```python
from build123d import *

# Parameters (mm, degrees)
SKETCH1_R           = 0.85
BOSS_EXTRUDE1_DEPTH = 3


with BuildPart() as part:
    # Sketch1 → Boss-Extrude1 (new body)
    with BuildSketch(Plane.XY):
        with BuildLine():
            Line((2.012075091, 4.025115381), (3.394482569, 4.82324871))
            Line((3.394482569, 4.82324871), (4.160527012, 4.1804611))
            Line((4.160527012, 4.1804611), (3.614571661, 2.6804611))
            ThreePointArc((3.614571661, 2.6804611), (3.897114317, 2.25), (4.128633237, 1.790080332))
            Line((4.128633237, 1.790080332), (5.700649018, 1.512891535))
            Line((5.700649018, 1.512891535), (5.874297196, 0.528083782))
            Line((5.874297196, 0.528083782), (4.491889718, -0.270049547))
            ThreePointArc((4.491889718, -0.270049547), (4.431634889, -0.7814168), (4.313358007, -1.282553199))
            Line((4.313358007, -1.282553199), (5.339418436, -2.505364402))
            Line((5.339418436, -2.505364402), (4.839418436, -3.371389806))
            Line((4.839418436, -3.371389806), (3.267402655, -3.09420101))
            ThreePointArc((3.267402655, -3.09420101), (2.892544244, -3.447199994), (2.479814627, -3.755065834))
            Line((2.479814627, -3.755065834), (2.479814627, -5.351332492))
            Line((2.479814627, -5.351332492), (1.540122006, -5.693352636))
            Line((1.540122006, -5.693352636), (0.514061576, -4.470541432))
            ThreePointArc((0.514061576, -4.470541432), (0, -4.5), (-0.514061576, -4.470541432))
            Line((-0.514061576, -4.470541432), (-1.540122006, -5.693352636))
            Line((-1.540122006, -5.693352636), (-2.479814627, -5.351332492))
            Line((-2.479814627, -5.351332492), (-2.479814627, -3.755065834))
            ThreePointArc((-2.479814627, -3.755065834), (-2.892544244, -3.447199994), (-3.267402655, -3.09420101))
            Line((-3.267402655, -3.09420101), (-4.839418436, -3.371389806))
            Line((-4.839418436, -3.371389806), (-5.339418436, -2.505364402))
            Line((-5.339418436, -2.505364402), (-4.313358007, -1.282553199))
            ThreePointArc((-4.313358007, -1.282553199), (-4.431634889, -0.7814168), (-4.491889718, -0.270049547))
            Line((-4.491889718, -0.270049547), (-5.874297196, 0.528083782))
            Line((-5.874297196, 0.528083782), (-5.700649018, 1.512891535))
            Line((-5.700649018, 1.512891535), (-4.128633237, 1.790080332))
            ThreePointArc((-4.128633237, 1.790080332), (-3.897114317, 2.25), (-3.614571661, 2.6804611))
            Line((-3.614571661, 2.6804611), (-4.160527012, 4.1804611))
            Line((-4.160527012, 4.1804611), (-3.394482569, 4.82324871))
            Line((-3.394482569, 4.82324871), (-2.012075091, 4.025115381))
            ThreePointArc((-2.012075091, 4.025115381), (-1.539090645, 4.228616794), (-1.045955351, 4.376754209))
            Line((-1.045955351, 4.376754209), (-0.5, 5.876754209))
            Line((-0.5, 5.876754209), (0.5, 5.876754209))
            Line((0.5, 5.876754209), (1.045955351, 4.376754209))
            ThreePointArc((1.045955351, 4.376754209), (1.539090645, 4.228616794), (2.012075091, 4.025115381))
        make_face()
        Circle(SKETCH1_R, mode=Mode.SUBTRACT)
    extrude(amount=BOSS_EXTRUDE1_DEPTH)


solid = part.part
```
Model file for the job. Use its own axes, mm. A direction names the side the tool comes from. Round coordinates to 2 decimals unless told otherwise and drop trailing zeros. Write each loop counter-clockwise with the first axis right and the second up, starting at its lowest first coordinate (ties: lowest second). Pieces come first, ordered by that corner, then holes. Notation, with made-up numbers: (71.5, 83) - (127.5, 83) arc R16 ccw to (127.5, 112) - close; hole circle Ø1 at (9.25, 63). An arc over 180 degrees is marked (long way). Use CSV: the item, a comma, the result in double quotes. Start each with the question number.
Item 1: Band-saw the part on B-B (y = 0). Write the cut outline in (x, z), and give its area (3 significant figures).
Item 2: Two-plate mould, pull along Y, no slides. Class faces 1 (the face through (-5.17, 0.12, 1.48)), 2 (the face through (-1.02, -5.073, 1.479)), 3 (the face through (-2.48, -5, 1)), 4 (the face through (-2.71, 4.43, 1.48)): released by +Y, released by -Y, zero draft, split by the parting line, or undercut.
Item 3: Tool access for faces 5 (the face through (3.89, 2.26, 1.48)), 6 (the face through (-3.884, 3.42, 1.479)), 7 (the face through (-1.546, 4.226, 1.479)), 8 (the face through (4.064, -3.235, 1.479)): list every direction of +Z, -Z, +X, -X, +Y, -Y with a clear straight run to the whole face (end or side of a thin tool).
Item 4: Band-saw the part on A-A (x = 0). Write the cut outline in (y, z), and give its area (3 significant figures).
Item 5: Drill centre lines: L1, parallel to Y at x = -5, z = 1.5; L2, parallel to X at y = 3, z = 0.75; L3, parallel to X at y = 3.25, z = 1.7. Where is each one in solid material? Low to high. Write a range as [from, to].
Item 6: Band-saw the part on C-C (y = 3.5). Write the cut outline in (x, z), and give its area (3 significant figures).
Item 7: Band-saw the part on D-D (x = 1.25). Write the cut outline in (y, z).
Item 8: Pin check, flat tips, straight feed: P1, Ø0.8, axis at y = -4.5, z = 1.5, coming from the +X side; P2, Ø0.5, axis at y = -4.5, z = 2, coming from the -X side; P3, Ø1, axis at x = 0, y = 0, coming from the -Z side. Stop position of each tip, or through.
Checked values:
1,outline,"(-4.96, 0) - (-0.85, 0) - (-0.85, 3) - (-4.96, 3) - close; (0.85, 0) - (4.96, 0) - (4.96, 3) - (0.85, 3) - close"
1,area,"24.7 mm²"
2,face 1,"undercut"
2,face 2,"released by -Y"
2,face 3,"zero draft"
2,face 4,"released by +Y"
3,face 5,"+Z, -Z, +X"
3,face 6,"+Z, -Z, -X"
3,face 7,"+Z, -Z, +Y"
3,face 8,"+Z, -Z, -Y"
4,outline,"(-4.5, 0) - (-0.85, 0) - (-0.85, 3) - (-4.5, 3) - close; (0.85, 0) - (5.88, 0) - (5.88, 3) - (0.85, 3) - close"
4,area,"26.0 mm²"
5,L1,"y = [-3.09, -2.1], [0.02, 1.64]"
5,L2,"x = [-3.73, 3.73]"
5,L3,"x = [-3.82, 3.82]"
6,outline,"(-3.91, 0) - (3.91, 0) - (3.91, 3) - (-3.91, 3) - close"
6,area,"23.5 mm²"
7,outline,"(-5.35, 0) - (4.32, 0) - (4.32, 3) - (-5.35, 3) - close"
8,P1,"stops at x = 2.48"
8,P2,"stops at x = -2.48"
8,P3,"passes through"
